from build123d import *
from build123d.topology import SkipClean

# Parameters (mm, degrees)
EXTRUDE_1_DEPTH          = 2
EXTRUDE_START            = -2
SKETCH_1_4_R             = 4.5
EXTRUDE_2_DEPTH          = 2
CUT_EXTRUDE_1_DEPTH      = 42.194659848
CUT_EXTRUDE_1_DEPTH_BACK = 42.194659848
SKETCH_1_3_R             = 2


with BuildPart() as part:
    # Sketch 1 → Extrude 1 (new body)
    with BuildSketch(Plane(origin=(0, 0, 0), x_dir=(0, 0, -1), z_dir=(1, 0, 0))):
        with BuildLine():
            Line((17.285303139, -16.066590839), (8.285303139, -2.066590839))
            ThreePointArc((8.285303139, -2.066590839), (3.231903814, -0.182369624), (0, -4.5))
            Line((0, -4.5), (0, -32.499999989))
            ThreePointArc((0, -32.499999989), (3.231903809, -36.817630374), (8.285303139, -34.933409161))
            Line((8.285303139, -34.933409161), (17.285303139, -20.933409161))
            ThreePointArc((17.285303139, -20.933409161), (18, -18.5), (17.285303139, -16.066590839))
        make_face()
    extrude(amount=EXTRUDE_1_DEPTH)

    # Sketch 1_4 → Extrude 2 (add)
    with SkipClean():  # the faces are left unmerged after this step: merging them gives an invalid solid
        with BuildSketch(Plane(origin=(0, 0, 0), x_dir=(0, 0, -1), z_dir=(1, 0, 0)).offset(EXTRUDE_START)):
            with Locations(Location((4.5, -4.5, 0), (0, 0, 180))):
                Circle(SKETCH_1_4_R)
        extrude(amount=EXTRUDE_2_DEPTH)

    # Sketch 1_3 → Cut-Extrude 1 (cut, two sides: drawn at the far end of the back side and taken through both)
    with SkipClean():  # the faces are left unmerged after this step: merging them gives an invalid solid
        with BuildSketch(Plane(origin=(0, 0, 0), x_dir=(0, 0, -1), z_dir=(1, 0, 0)).offset(-CUT_EXTRUDE_1_DEPTH_BACK)):
            with Locations((4.5, -4.5)):
                Circle(SKETCH_1_3_R)
            with Locations((13.5, -18.5)):
                Circle(SKETCH_1_3_R)
            with Locations((4.5, -32.5)):
                Circle(SKETCH_1_3_R)
        extrude(amount=CUT_EXTRUDE_1_DEPTH + CUT_EXTRUDE_1_DEPTH_BACK, mode=Mode.SUBTRACT)


solid = part.part
Design review of the part built by this model. Coordinates are the model's own, in mm. Round coordinates to 2 decimals unless told otherwise and drop trailing zeros. Loops run counter-clockwise (first coordinate to the right, second up) from the corner with the lowest first, then second, coordinate; pieces in that order, holes last. Notation, with made-up numbers: M -33.75,40.25 L 18.25,40.25 A18 cw 18.25,48.25 Z; hole C -2.75,57.5 d5. An arc over 180 degrees is marked long. Answer as a JSON object with one key per item and string values.
Item 1: The part is to be moulded in two halves that separate along Y. For faces 1 (the flat face through (0, -19, -7)), 2 (the cylindrical face through (0.986, -34.452, -4.066)), 3 (the cylindrical face through (0.986, -36.794, -3.154)), say which applies: pulls with the +Y half, pulls with the -Y half, needs draft (parallel to the pull), parting line crosses it, or undercut.
Answer sheet:
{"face 1": "needs draft", "face 2": "undercut", "face 3": "pulls with the -Y half"}
Item 2: We need section A-A on y = -18.5. Give the boundary of the cut face in (x, z), and give its area (3 significant figures).
Answer sheet:
{"outline": "M 0,-18 L 2,-18 L 2,-15.5 L 0,-15.5 Z; M 0,-11.5 L 2,-11.5 L 2,0 L 0,0 Z", "area": "28.0 mm^2"}
Item 3: Clearance check with a flat-ended pin moving along its axis: P1, Ø4.5, axis at y = -32.5, z = -4.5, coming from the -X side. State where the tip first meets the part, or that it passes through.
Answer sheet:
{"P1": "stops at x = 0"}
Item 4: We need section C-C on z = -15. Give the boundary of the cut face in (x, y), and give its area (3 significant figures).
Answer sheet:
{"outline": "M 0,-24.49 L 2,-24.49 L 2,-19.82 L 0,-19.82 Z; M 0,-17.18 L 2,-17.18 L 2,-12.51 L 0,-12.51 Z", "area": "18.7 mm^2"}
Item 5: We need section B-B on x = 0.5. Give the boundary of the cut face in (y, z).
Answer sheet:
{"outline": "M -34.93,-8.29 L -20.93,-17.29 A4.5 ccw -16.07,-17.29 L -2.07,-8.29 A4.5 ccw -4.5,0 L -32.5,0 A4.5 ccw Z; hole C -32.5,-4.5 d4; hole C -18.5,-13.5 d4; hole C -4.5,-4.5 d4"}
Item 6: Wall thickness on L1, parallel to Y at x = 1.4, z = -4.5; L2, parallel to Z at x = 1.75, y = -18.5; L3, parallel to Y at x = -1, z = -4.5: over which ranges is each line inside the solid? List them lowest first. Write a range as from..to.
Answer sheet:
{"L1": "y = -37..-34.5, -30.5..-6.5, -2.5..0", "L2": "z = -18..-15.5, -11.5..0", "L3": "y = -9..-6.5, -2.5..0"}
Item 7: We need section D-D on z = -4.5. Give the boundary of the cut face in (x, y).
Answer sheet:
{"outline": "M -2,-9 L 0,-9 L 0,-30.5 L 2,-30.5 L 2,-6.5 L -2,-6.5 Z; M -2,-2.5 L 2,-2.5 L 2,0 L -2,0 Z; M 0,-37 L 2,-37 L 2,-34.5 L 0,-34.5 Z"}
